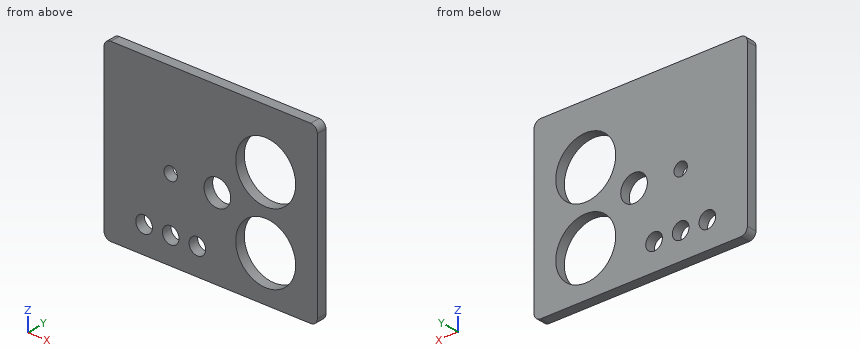
```python
from build123d import *

# Parameters (mm, degrees)
F1_DEPTH = 9.525
F2_R     = 28.575
F3_R     = 7.9375
F5_R     = 6.35
F4_R     = 12.7
F6_DEPTH = 9.526


with BuildPart() as f1:
    # F0 (on Front) → F1 (new body)
    with BuildSketch(Plane.XZ):
        with BuildLine():
            Line((-95.25, -82.55), (95.25, -82.55))
            ThreePointArc((95.25, -82.55), (99.740128, -80.690128), (101.6, -76.2))
            Line((101.6, -76.2), (101.6, 76.2))
            ThreePointArc((101.6, 76.2), (99.740128, 80.690128), (95.25, 82.55))
            Line((95.25, 82.55), (-95.25, 82.55))
            ThreePointArc((-95.25, 82.55), (-99.740128, 80.690128), (-101.6, 76.2))
            Line((-101.6, 76.2), (-101.6, -76.2))
            ThreePointArc((-101.6, -76.2), (-99.740128, -80.690128), (-95.25, -82.55))
        make_face()
    extrude(amount=F1_DEPTH)

    # F2 (on face) + F3 (on face) + F5 (on face) + F4 (on face) → F6 (cut, through all)
    with BuildSketch(Plane.XZ.offset(9.525)):
        with Locations((52.3875, 26.9875)):
            Circle(F2_R)
        with Locations((52.3875, -39.6875)):
            Circle(F2_R)
    with BuildSketch(Plane.XZ.offset(9.525)):
        with Locations((-63.5, -57.15)):
            Circle(F3_R)
        with Locations((-38.1, -57.15)):
            Circle(F3_R)
        with Locations((-12.7, -57.15)):
            Circle(F3_R)
    with BuildSketch(Plane.XZ.offset(9.525)):
        with Locations((-38.1, -6.35)):
            Circle(F5_R)
    with BuildSketch(Plane.XZ.offset(9.525)):
        with Locations((6.35, -6.35)):
            Circle(F4_R)
    extrude(amount=-F6_DEPTH, mode=Mode.SUBTRACT)


solid = f1.part
```
For this review, take the finished solid that the model builds, in its own axes (mm). Give positions to 0.01 mm unless a question says otherwise; leave off trailing zeros. Order: outer loops, then holes, each group sorted by start corner. A loop starts at its lowest first (then second) coordinate and runs counter-clockwise, first axis right, second up.
1) Take a section at B-B (z = 23.5). Give the boundary of the cut face in (x, y) (3 decimals).
2) Take a section at A-A (x = -38.1). State how many separate pieces and enclosed holes the cut face has, then the cut area to 3 significant figures.
3) Insertion check: pin 1 (9.5 mm diameter, centred on x = -38.1, z = -57.15, fed in from -Y). The pin has a flat end and moves straight along its axis. Give the tip position at first contact, or say it passes through.
4) Take a section at C-C (z = -6.35). Give the boundary of the cut face in (x, y) (3 decimals), then the cut area to 3 significant figures.
5) Take a section at D-D (x = 15.5). Give the boundary of the cut face in (y, z) (3 decimals), then the cut area to 3 significant figures.
6) Wall thickness on line 1 (Z direction, x = -38.1, y = -3.5); line 2 (Z direction, x = 53.5, y = -6.25); line 3 (Z direction, x = -12.7, y = -3.75): over which ranges is each line inside the solid? List them lowest first.
Derived:
1. outline: (-101.6, -9.525) - (24.026, -9.525) - (24.026, 0) - (-101.6, 0) - close; (80.749, -9.525) - (101.6, -9.525) - (101.6, 0) - (80.749, 0) - close
2. separate pieces: 3
2. enclosed holes: 0
2. area: 1,300 mm2
3. pin 1: passes through
4. outline: (-101.6, -9.525) - (-44.45, -9.525) - (-44.45, 0) - (-101.6, 0) - close; (-31.75, -9.525) - (-6.35, -9.525) - (-6.35, 0) - (-31.75, 0) - close; (19.05, -9.525) - (101.6, -9.525) - (101.6, 0) - (19.05, 0) - close
4. area: 1,570 mm2
5. outline: (-9.525, -82.55) - (0, -82.55) - (0, -15.157) - (-9.525, -15.157) - close; (-9.525, 2.457) - (0, 2.457) - (0, 82.55) - (-9.525, 82.55) - close
5. area: 1,400 mm2
6. line 1: z = -82.55 to -65.09, -49.21 to -12.7, 0 to 82.55
6. line 2: z = -82.55 to -68.24, -11.13 to -1.57, 55.54 to 82.55
6. line 3: z = -82.55 to -65.09, -49.21 to 82.55
